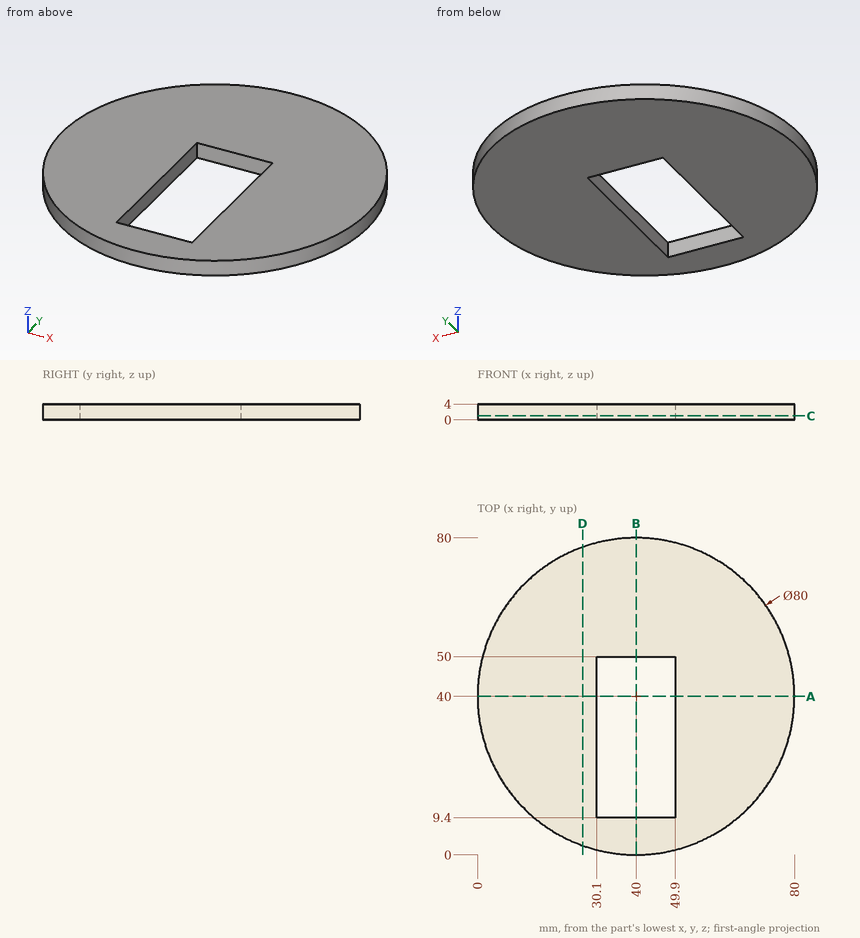
Study the drawing (mm; zero at the part's minimum x, y, z) and answer. Coordinates: 2 decimals unless noted, no trailing zeros. Loops run counter-clockwise (first coordinate to the right, second up) from the corner with the lowest first, then second, coordinate; pieces in that order, holes last. Notation, with made-up numbers: (37.5, 24) -> (47.5, 24) arc R32 ccw to (47.5, 63) -> close; hole circle Ø6 at (-25.75, 39). An arc over 180 degrees is marked (long way). Answer as CSV lines item,"result".
1) The part is cut by section C-C (z = 1). Give the vertices of the cut face in (x, y), and give its area (3 significant figures).
A:
outline,"circle Ø80 at (40, 40); hole (30.1, 9.4) -> (49.9, 9.4) -> (49.9, 50) -> (30.1, 50) -> close"
area,"4,220 mm²"
2) The part is cut by section B-B (x = 40). Give the vertices of the cut face in (y, z).
A:
outline,"(0, 0) -> (9.4, 0) -> (9.4, 4) -> (0, 4) -> close; (50, 0) -> (80, 0) -> (80, 4) -> (50, 4) -> close"
3) The part is cut by section A-A (y = 40). Give the vertices of the cut face in (x, z).
A:
outline,"(0, 0) -> (30.1, 0) -> (30.1, 4) -> (0, 4) -> close; (49.9, 0) -> (80, 0) -> (80, 4) -> (49.9, 4) -> close"
4) The part is cut by section D-D (x = 26.5). Give the vertices of the cut face in (y, z).
A:
outline,"(2.35, 0) -> (77.65, 0) -> (77.65, 4) -> (2.35, 4) -> close"
5) Straight lines are drawn through the part: probe 1 along X at (y, z) = (10, 1.4); probe 2 along Y at (x, z) = (46, 0.4); probe 3 along X at (y, z) = (47, 3.55). For each, find the intervals that lie inside material, in ascending order.
A:
probe 1,"x = 13.54 to 30.1, 49.9 to 66.46"
probe 2,"y = 0.45 to 9.4, 50 to 79.55"
probe 3,"x = 0.62 to 30.1, 49.9 to 79.38"
6) Flat-ended cylindrical pins translate along their axes: pin 1 (1.2 mm diameter, centred on x = 40.5, z = 2, fed in from +Y); pin 2 (1 mm diameter, centred on x = 43.5, z = 2, fed in from +Y). Find the tip coordinate at first contact, or state that the pin passes through.
A:
pin 1,"stops at y = 80"
pin 2,"stops at y = 79.89"
